CAD build for the part. Positions are in the model's coordinates, mm. A direction names the side the tool comes from. Give positions to 0.01 mm unless a question says otherwise; leave off trailing zeros. Write each loop counter-clockwise with the first axis right and the second up, starting at its lowest first coordinate (ties: lowest second). Pieces come first, ordered by that corner, then holes. Notation, with made-up numbers: M -34.75,60 L 9.25,60 A3 cw 9.25,65 Z; hole C -2.5,-37.75 d2. An arc over 180 degrees is marked long. One line per question, with ' | ' between items. Start each with the question number.
1. Cut at D-D, the plane z = 47.5. Write the cut outline in (x, y).
2. Flat gauge pins, fed straight in: pin 1 (1 mm diameter, centred on x = 539, y = -73.5, fed in from -Z); pin 2 (4 mm diameter, centred on x = 622, z = 69.5, fed in from -Y); pin 3 (3 mm diameter, centred on x = 456, z = -16, fed in from -Y). Where does each tip first touch, or does it go through?
3. Cut at A-A, the plane y = -117.5. Write the cut outline in (x, z).
4. Cut at C-C, the plane x = 580.5. Write the cut outline in (y, z), then the cut area to 3 significant figures.
5. Which spindle directions (+Z, -Z, +X, -X, +Y, -Y) get a long thin tool onto all of the face, cutting with end or side? Do faces 4 (the face through (609.6, -106, -2)), 5 (the face through (762, -58, -2)). Say none if no direction does.
6. Cut at B-B, the plane z = 103. Write the cut outline in (x, y).
7. Wall check: L1, parallel to X at y = -109.5, z = 47.5; L2, parallel to Y at x = 343.5, z = -57; L3, parallel to Y at x = 692, z = -4. Give the ranges that are in metal, low to high.
8. Pull direction X, two halves, no side cores. Call faces 1 (the face through (152.4, -58, -2)), 2 (the face through (453, 0, -2)), 3 (the face through (455, -76.2, -2)): released by +X, released by -X, zero draft, split by the parting line, or undercut.
```python
from build123d import *

# Parameters (mm, degrees)
BASE_DEPTH      = 914.4
SLOT_DEPTH      = 940.456694052
SLOT_DEPTH_BACK = 940.456694052
SKETCH2_W       = 304.8
SKETCH2_H       = 76.2
LEFT_CUT_DEPTH  = 152.4


with BuildPart() as part:
    # Sketch1 → Base (new body)
    with BuildSketch(Plane(origin=(0, 0, 0), x_dir=(0, 0, -1), z_dir=(1, 0, 0))):
        with BuildLine():
            Line((152.4, 0), (-152.4, 0))
            ThreePointArc((-152.4, 0), (0, -152.4), (152.4, 0))
        make_face()
    extrude(amount=BASE_DEPTH)

    # Sketch2 → Slot (cut, two sides: drawn at the far end of the back side and taken through both)
    with BuildSketch(Plane.XY.offset(-SLOT_DEPTH_BACK)):
        with Locations((457.2, -114.3)):
            Rectangle(SKETCH2_W, SKETCH2_H)
    extrude(amount=SLOT_DEPTH + SLOT_DEPTH_BACK, mode=Mode.SUBTRACT)

    # Sketch3 → Left Cut (cut)
    with BuildSketch(Plane.ZY):
        with BuildLine():
            Line((152.4, 0), (-152.4, 0))
            ThreePointArc((-152.4, 0), (0, -152.4), (152.4, 0))
        make_face()
    left_cut = extrude(amount=-LEFT_CUT_DEPTH, mode=Mode.SUBTRACT)

    # Right Cut: Left Cut across plane
    add(left_cut.mirror(Plane(origin=(457.2, 0, 0), x_dir=(0, 0, 1), z_dir=(1, 0, 0))), mode=Mode.SUBTRACT)


solid = part.part
```
Here are the results:
1) outline: M 152.4,-144.81 L 304.8,-144.81 L 304.8,-76.2 L 609.6,-76.2 L 609.6,-144.81 L 762,-144.81 L 762,0 L 152.4,0 Z
2) pin 1: z = -133.78 | pin 2: y = -136.64 | pin 3: y = -76.2
3) outline: M 152.4,-97.05 L 304.8,-97.05 L 304.8,97.05 L 152.4,97.05 Z; M 609.6,-97.05 L 762,-97.05 L 762,97.05 L 609.6,97.05 Z
4) outline: M -76.2,-131.98 A152.4 ccw 0,-152.4 L 0,152.4 A152.4 ccw -76.2,131.98 Z | area: 22,200 mm^2
5) face 4: +Z, -Z, -Y | face 5: +Z, -Z, +X, +Y, -Y
6) outline: M 152.4,-112.32 L 304.8,-112.32 L 304.8,-76.2 L 609.6,-76.2 L 609.6,-112.32 L 762,-112.32 L 762,0 L 152.4,0 Z
7) L1: 152.4 to 304.8, 609.6 to 762 | L2: -76.2 to 0 | L3: -152.35 to 0
8) face 1: released by -X | face 2: zero draft | face 3: undercut
